from build123d import *

# Parameters (mm, degrees)
BOSS_EXTRUDE1_DEPTH          = 12.7
SKETCH2_R                    = 1.5875
SIDE_MOUNT_HOLES_DEPTH       = 12.7
SKETCH3_R                    = 1.5875
TOP_BOTTOM_MOUNT_HOLES_DEPTH = 12.7
FILLET1_R                    = 2.54
FILLET2_R                    = 5.08
FILLET3_R                    = 1.27


with BuildPart() as part:
    # Sketch1 → Boss-Extrude1 (new body)
    with BuildSketch(Plane(origin=(0, 0, 0), x_dir=(0, 0, -1), z_dir=(1, 0, 0))):
        Polygon((0, 0), (-19.05, 0), (-19.05, 3.81), (-6.35, 3.81), (-6.35, 95.25), (-133.35, 95.25), (-133.35, 82.55), (-137.16, 82.55), (-137.16, 120.65), (-133.35, 120.65), (-133.35, 107.95), (-6.35, 107.95), (-6.35, 186.436), (-19.05, 186.436), (-19.05, 190.246), (19.05, 190.246), (19.05, 186.436), (6.35, 186.436), (6.35, 3.81), (19.05, 3.81), (19.05, 0), align=None)
    extrude(amount=BOSS_EXTRUDE1_DEPTH)

    # Sketch2 → Side_mount_holes (cut)
    with BuildSketch(Plane.XY.offset(137.16)):
        with Locations((6.35, 114.3)):
            Circle(SKETCH2_R)
        with Locations(Location((6.35, 88.9, 0), (0, 0, 270))):
            Circle(SKETCH2_R)
    extrude(amount=-SIDE_MOUNT_HOLES_DEPTH, mode=Mode.SUBTRACT)

    # Sketch3 → top_Bottom_mount_holes (cut)
    with BuildSketch(Plane.XZ):
        with Locations(Location((6.35, 12.7, 0), (0, 0, 270))):
            Circle(SKETCH3_R)
        with Locations(Location((6.35, -12.7, 0), (0, 0, 270))):
            Circle(SKETCH3_R)
    top_bottom_mount_holes = extrude(amount=-TOP_BOTTOM_MOUNT_HOLES_DEPTH, mode=Mode.SUBTRACT)

    # Mirror1: top_Bottom_mount_holes across plane
    add(top_bottom_mount_holes.mirror(Plane(origin=(0, 95.123, 0), x_dir=(0, 0, 1), z_dir=(0, -1, 0))), mode=Mode.SUBTRACT)

    # Fillet1
    fillet1_edges = [part.edges().sort_by_distance(p)[0] for p in [
        (6.35, 3.81, 6.35),
        (6.35, 95.25, 133.35),
        (6.35, 107.95, 133.35),
        (6.35, 186.436, 6.35),
        (6.35, 186.436, -6.35),
        (6.35, 3.81, -6.35),
    ]]
    fillet(fillet1_edges, radius=FILLET1_R)

    # Fillet2
    fillet2_edges = [part.edges().sort_by_distance(p)[0] for p in [
        (6.35, 95.25, 6.35),
        (6.35, 107.95, 6.35),
    ]]
    fillet(fillet2_edges, radius=FILLET2_R)

    # Fillet3
    fillet3_edges = [part.edges().sort_by_distance(p)[0] for p in [
        (6.35, 0, 19.05),
        (6.35, 3.81, 19.05),
        (6.35, 82.55, 133.35),
        (6.35, 82.55, 137.16),
        (6.35, 120.65, 137.16),
        (6.35, 120.65, 133.35),
        (6.35, 186.436, 19.05),
        (6.35, 190.246, 19.05),
        (6.35, 190.246, -19.05),
        (6.35, 186.436, -19.05),
        (6.35, 3.81, -19.05),
        (6.35, 0, -19.05),
    ]]
    fillet(fillet3_edges, radius=FILLET3_R)


solid = part.part
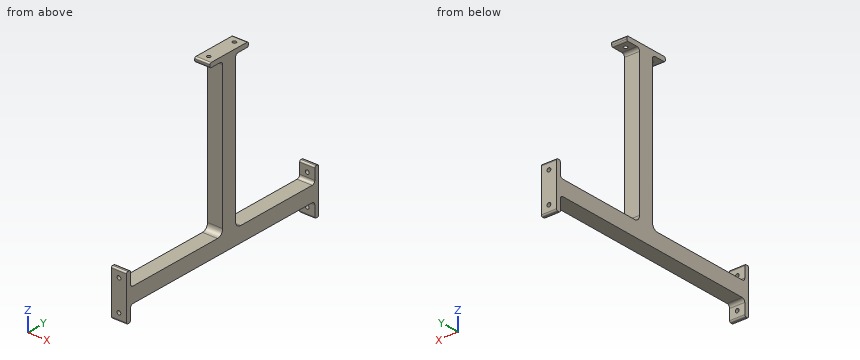
Read the model definition and answer for the solid it produces. Units are mm, in the model's axes. Give positions to 0.01 mm unless a question says otherwise; leave off trailing zeros. Write each loop counter-clockwise with the first axis right and the second up, starting at its lowest first coordinate (ties: lowest second). Pieces come first, ordered by that corner, then holes. Notation, with made-up numbers: (-24.5, 49.5) - (9.5, 49.5) arc R20 cw to (9.5, 71.5) - close; hole circle Ø3 at (83, 71.25). An arc over 180 degrees is marked (long way). Return JSON: item names as keys, results as strings.
Q1. A cutting plane is placed at A-A, the plane z = 33. Determine the outline of the cut face in (x, y).
Reply:
{"outline": "(0, 95.25) - (12.7, 95.25) - (12.7, 107.95) - (0, 107.95) - close"}
Q2. Given P1, Ø4, axis at x = 6.5, z = 116.5, coming from the +Y side; P2, Ø2.5, axis at x = 6.35, y = 88.9, coming from the +Z side; P3, Ø1, axis at x = 7, z = 135, coming from the +Y side, each flat-ended and moving along its own axis, determine where each tip first touches the part or whether it passes through.
Reply:
{"P1": "y = 107.95", "P2": "z = 6.35", "P3": "y = 120.65"}
Q3. Consider line 1 along Y through (x, z) = (8.5, 17.5); line 2 along Y through (x, z) = (8.5, 18); line 3 along Y through (x, z) = (6.25, -11). Determine where each line is inside the solid, lowest interval first. Write a range as [from, to].
Reply:
{"line 1": "[0, 3.81], [95.25, 107.95], [186.44, 190.25]", "line 2": "[0.02, 3.79], [95.25, 107.95], [186.46, 190.23]", "line 3": "[0, 3.81], [186.44, 190.25]"}
Q4. A cutting plane is placed at B-B, the plane y = 102.5. Determine the outline of the cut face in (x, z).
Reply:
{"outline": "(0, -6.35) - (12.7, -6.35) - (12.7, 137.16) - (0, 137.16) - close"}
